Geometry check sheet. Reference: the model listing, model coordinates, mm. Face numbers are marked on the shaded views. Coordinates: 2 decimals unless noted, no trailing zeros. Order: outer loops, then holes, each group sorted by start corner. A loop starts at its lowest first (then second) coordinate and runs counter-clockwise, first axis right, second up. Notation, with made-up numbers: (2, 44) - (8, 44) arc R16 ccw to (8, 70) - close; hole circle Ø5 at (19, 27). An arc over 180 degrees is marked (long way). Use CSV: the item, a comma, the result in double quotes. Start each with the question number.
1) Draft check along Z on the marked faces 1, 2 and 3. Enter one of: released by +Z, released by -Z, zero draft, split by the parting line, or undercut.
2) Sectioned sample at A-A, the plane x = 0. Record the cut outline in (y, z).
3) Depth check by flat-ended pin: P1, Ø5, axis at x = 85.5, z = -49, coming from the +Y side; P2, Ø5.5, axis at x = 0, z = 95.25, coming from the +Y side; P3, Ø8, axis at x = -50.5, y = -33.5, coming from the +Z side; P4, Ø12, axis at x = -34.5, y = -50.5, coming from the +Z side. Enter the tip coordinate at first touch or a pass-through.
4) Sectioned sample at C-C, the plane x = 95.25. Record the cut outline in (y, z).
5) Sectioned sample at B-B, the plane z = 0. Record the cut outline in (x, y), and give its area (3 significant figures).
6) Thickness scan on probe 1 along X at (y, z) = (-79.05, 0); probe 2 along X at (y, z) = (32, 0). Record the ranges inside material, lowest first. Write a range as [from, to].
7) Sectioned sample at D-D, the plane y = -57. Record the cut outline in (x, z), and give its area (3 significant figures).
from build123d import *

# Parameters (mm, degrees)
CUT_EXTRUDE2_REACH = 228.224
MOTOR_HOLE_R       = 25.4
MOTOR_HOLE_R_2     = 4.7625


with BuildPart() as part:
    # Compartment → Revolve1 (revolve)
    with BuildSketch(Plane.XY, mode=Mode.PRIVATE) as revolve1_sk:
        Polygon((115.189, -80), (0, -80), (0, -77.46), (112.649, -77.46), (112.649, 76.972), (115.189, 76.972), align=None)
    revolve(revolve1_sk.sketch.rotate(Axis((0, 0, 0), (0, 1, 0)), 90), axis=Axis((0, 0, 0), (0, 1, 0)))

    # Motor Hole → Cut-Extrude2 (cut, up to next)
    with BuildSketch(Plane.XZ.offset(80), mode=Mode.PRIVATE) as cut_extrude2_sk1:
        with Locations(Location((0, 0, 0), (0, 0, 270))):
            Circle(MOTOR_HOLE_R)
    cut_extrude2_tool1 = extrude(cut_extrude2_sk1.sketch, amount=-CUT_EXTRUDE2_REACH, mode=Mode.PRIVATE) & part.part
    # Motor Hole → Cut-Extrude2 (cut, up to next)
    with BuildSketch(Plane.XZ.offset(80), mode=Mode.PRIVATE) as cut_extrude2_sk2:
        with Locations(Location((0, 95.25, 0), (0, 0, 270))):
            Circle(MOTOR_HOLE_R_2)
    cut_extrude2_tool2 = extrude(cut_extrude2_sk2.sketch, amount=-CUT_EXTRUDE2_REACH, mode=Mode.PRIVATE) & part.part
    # Motor Hole → Cut-Extrude2 (cut, up to next)
    with BuildSketch(Plane.XZ.offset(80), mode=Mode.PRIVATE) as cut_extrude2_sk3:
        with Locations(Location((95.25, 0, 0), (0, 0, 270))):
            Circle(MOTOR_HOLE_R_2)
    cut_extrude2_tool3 = extrude(cut_extrude2_sk3.sketch, amount=-CUT_EXTRUDE2_REACH, mode=Mode.PRIVATE) & part.part
    # Motor Hole → Cut-Extrude2 (cut, up to next)
    with BuildSketch(Plane.XZ.offset(80), mode=Mode.PRIVATE) as cut_extrude2_sk4:
        with Locations(Location((0, -95.25, 0), (0, 0, 270))):
            Circle(MOTOR_HOLE_R_2)
    cut_extrude2_tool4 = extrude(cut_extrude2_sk4.sketch, amount=-CUT_EXTRUDE2_REACH, mode=Mode.PRIVATE) & part.part
    # Motor Hole → Cut-Extrude2 (cut, up to next)
    with BuildSketch(Plane.XZ.offset(80), mode=Mode.PRIVATE) as cut_extrude2_sk5:
        with Locations(Location((-95.25, 0, 0), (0, 0, 270))):
            Circle(MOTOR_HOLE_R_2)
    cut_extrude2_tool5 = extrude(cut_extrude2_sk5.sketch, amount=-CUT_EXTRUDE2_REACH, mode=Mode.PRIVATE) & part.part
    add(cut_extrude2_tool1.solids().sort_by_distance((0, -80, 0))[0], mode=Mode.SUBTRACT)
    add(cut_extrude2_tool2.solids().sort_by_distance((0, -80, 95.25))[0], mode=Mode.SUBTRACT)
    add(cut_extrude2_tool3.solids().sort_by_distance((95.25, -80, 0))[0], mode=Mode.SUBTRACT)
    add(cut_extrude2_tool4.solids().sort_by_distance((0, -80, -95.25))[0], mode=Mode.SUBTRACT)
    add(cut_extrude2_tool5.solids().sort_by_distance((-95.25, -80, 0))[0], mode=Mode.SUBTRACT)


solid = part.part
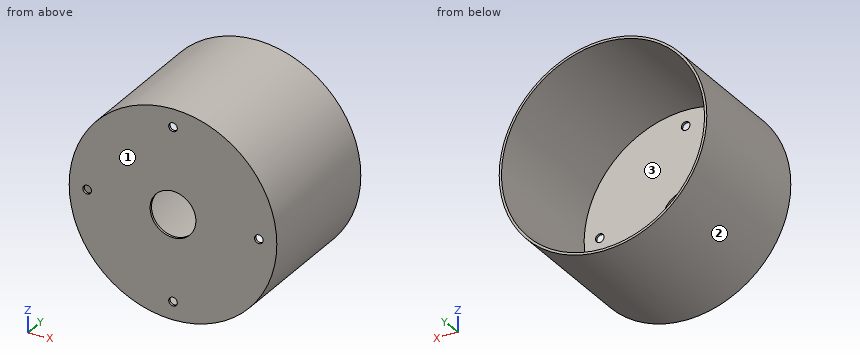
Evaluation:
1,face 1,"zero draft"
1,face 2,"split by the parting line"
1,face 3,"undercut"
2,outline,"(-80, -115.19) - (76.97, -115.19) - (76.97, -112.65) - (-77.46, -112.65) - (-77.46, -100.01) - (-80, -100.01) - close; (-80, -90.49) - (-77.46, -90.49) - (-77.46, -25.4) - (-80, -25.4) - close; (-80, 25.4) - (-77.46, 25.4) - (-77.46, 90.49) - (-80, 90.49) - close; (-80, 100.01) - (-77.46, 100.01) - (-77.46, 112.65) - (76.97, 112.65) - (76.97, 115.19) - (-80, 115.19) - close"
3,P1,"y = -77.46"
3,P2,"through"
3,P3,"z = 105.39"
3,P4,"z = 111.61"
4,outline,"(-80, -64.78) - (76.97, -64.78) - (76.97, -60.14) - (-77.46, -60.14) - (-77.46, -4.76) - (-80, -4.76) - close; (-80, 4.76) - (-77.46, 4.76) - (-77.46, 60.14) - (76.97, 60.14) - (76.97, 64.78) - (-80, 64.78) - close"
5,outline,"(-115.19, -80) - (-100.01, -80) - (-100.01, -77.46) - (-112.65, -77.46) - (-112.65, 76.97) - (-115.19, 76.97) - close; (-90.49, -80) - (-25.4, -80) - (-25.4, -77.46) - (-90.49, -77.46) - close; (25.4, -80) - (90.49, -80) - (90.49, -77.46) - (25.4, -77.46) - close; (100.01, -80) - (115.19, -80) - (115.19, 76.97) - (112.65, 76.97) - (112.65, -77.46) - (100.01, -77.46) - close"
5,area,"1,190 mm²"
6,probe 1,"[-115.19, -100.01], [-90.49, -25.4], [25.4, 90.49], [100.01, 115.19]"
6,probe 2,"[-115.19, -112.65], [112.65, 115.19]"
7,outline,"circle Ø230.38 at (0, 0); hole circle Ø225.3 at (0, 0)"
7,area,"1,820 mm²"
